Geometry check sheet. Reference: the model listing, model coordinates, mm. Coordinates: 2 decimals unless noted, no trailing zeros. Write each loop counter-clockwise with the first axis right and the second up, starting at its lowest first coordinate (ties: lowest second). Pieces come first, ordered by that corner, then holes. Notation, with made-up numbers: (69.25, -14.5) -> (73.25, -14.5) arc R31 cw to (73.25, 9.5) -> close; hole circle Ø9 at (17, 60.25). An arc over 180 degrees is marked (long way). Answer in a Markdown table with one row per item. Add a question column.
1. Scan lines: L1, parallel to Z at x = -41, y = 0.5; L2, parallel to Z at x = -16, y = 1.75; L3, parallel to Z at x = -6, y = 0.75. Record each from-to range of solid material in increasing order. Write a range as from..to.
2. Depth check by flat-ended pin: P1, Ø5.5, axis at x = 46.23, z = -50.74, coming from the -Y side. Enter the tip coordinate at first touch or a pass-through.
3. Cross-section at A-A on x = -36.83. Record the cut outline in (y, z), and give its area (3 significant figures).
4. Cross-section at B-B on y = 2.25. Give the number of separate pieces and of enclosed holes in the cut face, and give its area (3 significant figures).
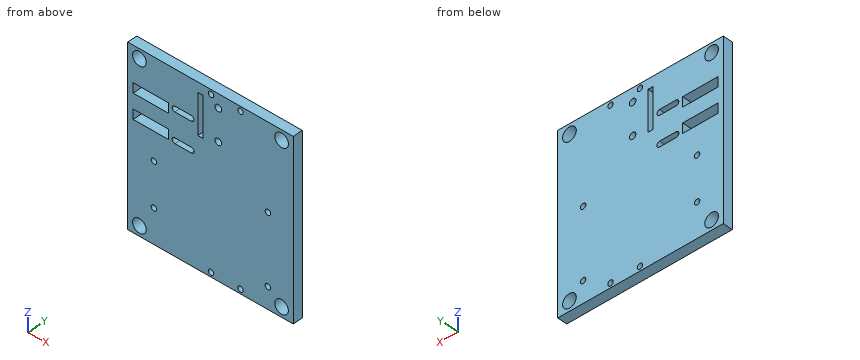
```python
from build123d import *

# Parameters (mm, degrees)
ESQUISSE1_W             = 107.696
ESQUISSE1_H             = 114.173
BOSS_EXTRU_1_DEPTH      = 6.35
ESQUISSE1_6_OUTSIDE_W   = 141.112
ESQUISSE1_6_OUTSIDE_H   = 147.588
ESQUISSE1_6_OUTSIDE_W_2 = 107.696
ESQUISSE1_6_OUTSIDE_H_2 = 114.173
ESQUISSE1_6_OUTSIDE_R   = 1.778
ESQUISSE1_6_OUTSIDE_R_2 = 4.445
ESQUISSE1_6_OUTSIDE_W_3 = 3.302
ESQUISSE1_6_OUTSIDE_H_3 = 25.4
ESQUISSE1_6_OUTSIDE_W_4 = 22.86
ESQUISSE1_6_OUTSIDE_H_4 = 6.35
ENL_V_MAT_EXTRU_3_DEPTH = 7.35
ESQUISSE2_R             = 1.778
BOSS_EXTRU_2_DEPTH      = 6.35
ESQUISSE3_R             = 2.135000048
ESQUISSE3_W             = 3.302
ESQUISSE3_H             = 0.79375
ENL_V_MAT_EXTRU_4_DEPTH = 7.35


with BuildPart() as part:
    # Esquisse1 → Boss.-Extru.1 (new body)
    with BuildSketch(Plane(origin=(0, 0, 0), x_dir=(1, 0, 0), z_dir=(0, 1, 0))):
        Rectangle(ESQUISSE1_W, ESQUISSE1_H)
    extrude(amount=BOSS_EXTRU_1_DEPTH)

    # Esquisse1<6> outside → Enlèv. mat.-Extru.3 (cut, through all)
    with BuildSketch(Plane(origin=(0, 0, 0), x_dir=(1, 0, 0), z_dir=(0, 1, 0))):
        Rectangle(ESQUISSE1_6_OUTSIDE_W, ESQUISSE1_6_OUTSIDE_H)
        Rectangle(ESQUISSE1_6_OUTSIDE_W_2, ESQUISSE1_6_OUTSIDE_H_2, mode=Mode.SUBTRACT)
        with Locations((0.3429, -54.1147)):
            Circle(ESQUISSE1_6_OUTSIDE_R)
        with Locations((19.5199, -54.1147)):
            Circle(ESQUISSE1_6_OUTSIDE_R)
        with Locations((6.858, -49.9745)):
            Circle(ESQUISSE1_6_OUTSIDE_R)
        with Locations((6.858, -30.6705)):
            Circle(ESQUISSE1_6_OUTSIDE_R)
        with Locations((-4.572, -23.0505)):
            Circle(ESQUISSE1_6_OUTSIDE_R)
        with Locations((46.228, -50.7365)):
            Circle(ESQUISSE1_6_OUTSIDE_R_2)
        with Locations((46.228, 50.7365)):
            Circle(ESQUISSE1_6_OUTSIDE_R_2)
        with Locations((37.338, 43.1165)):
            Circle(ESQUISSE1_6_OUTSIDE_R)
        with Locations((37.338, -2.0955)):
            Circle(ESQUISSE1_6_OUTSIDE_R)
        with Locations((-36.83, 34.8361)):
            Circle(ESQUISSE1_6_OUTSIDE_R)
        with Locations((-36.83, 6.2865)):
            Circle(ESQUISSE1_6_OUTSIDE_R)
        with Locations((19.5199, 54.1147)):
            Circle(ESQUISSE1_6_OUTSIDE_R)
        with Locations((0.3429, 54.1147)):
            Circle(ESQUISSE1_6_OUTSIDE_R)
        with Locations((-46.228, 50.7365)):
            Circle(ESQUISSE1_6_OUTSIDE_R_2)
        with Locations((-46.228, -50.9905)):
            Circle(ESQUISSE1_6_OUTSIDE_R_2)
        with Locations((-6.5278, -38.0365)):
            Rectangle(ESQUISSE1_6_OUTSIDE_W_3, ESQUISSE1_6_OUTSIDE_H_3)
        with Locations((-38.862, -15.0495)):
            Rectangle(ESQUISSE1_6_OUTSIDE_W_4, ESQUISSE1_6_OUTSIDE_H_4)
        with Locations((-38.862, -31.0515)):
            Rectangle(ESQUISSE1_6_OUTSIDE_W_4, ESQUISSE1_6_OUTSIDE_H_4)
        with BuildLine():
            Line((-23.1394, -34.4805), (-12.4714, -34.4805))
            ThreePointArc((-12.4714, -34.4805), (-10.6934, -32.7025), (-12.4714, -30.9245))
            Line((-12.4714, -30.9245), (-23.1394, -30.9245))
            ThreePointArc((-23.1394, -30.9245), (-24.9174, -32.7025), (-23.1394, -34.4805))
        make_face()
        with BuildLine():
            Line((-23.1394, -15.1765), (-12.4714, -15.1765))
            ThreePointArc((-12.4714, -15.1765), (-10.6934, -13.3985), (-12.4714, -11.6205))
            Line((-12.4714, -11.6205), (-23.1394, -11.6205))
            ThreePointArc((-23.1394, -11.6205), (-24.9174, -13.3985), (-23.1394, -15.1765))
        make_face()
    extrude(amount=ENL_V_MAT_EXTRU_3_DEPTH, mode=Mode.SUBTRACT)

    # Esquisse2 → Boss.-Extru.2 (add)
    with BuildSketch(Plane(origin=(0, 6.35, 0), x_dir=(1, 0, 0), z_dir=(0, 1, 0))):
        with Locations((-4.572, -23.0505)):
            Circle(ESQUISSE2_R)
        with Locations((6.858, -30.6705)):
            Circle(ESQUISSE2_R)
        with Locations((6.858, -49.9745)):
            Circle(ESQUISSE2_R)
    extrude(amount=-BOSS_EXTRU_2_DEPTH)

    # Esquisse3 → Enlèv. mat.-Extru.4 (cut, through all)
    with BuildSketch(Plane(origin=(0, 6.35, 0), x_dir=(1, 0, 0), z_dir=(0, 1, 0))):
        with Locations((5.0992, -27.7865)):
            Circle(ESQUISSE3_R)
        with Locations((5.0992, -48.2865)):
            Circle(ESQUISSE3_R)
        with Locations((-6.5278, -24.939625)):
            Rectangle(ESQUISSE3_W, ESQUISSE3_H)
    extrude(amount=-ENL_V_MAT_EXTRU_4_DEPTH, mode=Mode.SUBTRACT)


solid = part.part
```
Results found:
| question | item | result |
|---|---|---|
| 1 | L1 | z = -57.09..11.87, 18.22..27.88, 34.23..57.09 |
| 1 | L2 | z = -57.09..11.62, 15.18..30.92, 34.48..57.09 |
| 1 | L3 | z = -57.09..24.54, 50.74..57.09 |
| 2 | P1 | passes through |
| 3 | outline | (0, -57.09) -> (6.35, -57.09) -> (6.35, -36.61) -> (0, -36.61) -> close; (0, -33.06) -> (6.35, -33.06) -> (6.35, -8.06) -> (0, -8.06) -> close; (0, -4.51) -> (6.35, -4.51) -> (6.35, 11.87) -> (0, 11.87) -> close; (0, 18.22) -> (6.35, 18.22) -> (6.35, 27.88) -> (0, 27.88) -> close; (0, 34.23) -> (6.35, 34.23) -> (6.35, 57.09) -> (0, 57.09) -> close |
| 3 | area | 599 mm^2 |
| 4 | separate pieces | 1 |
| 4 | enclosed holes | 19 |
| 4 | area | 11,500 mm^2 |
